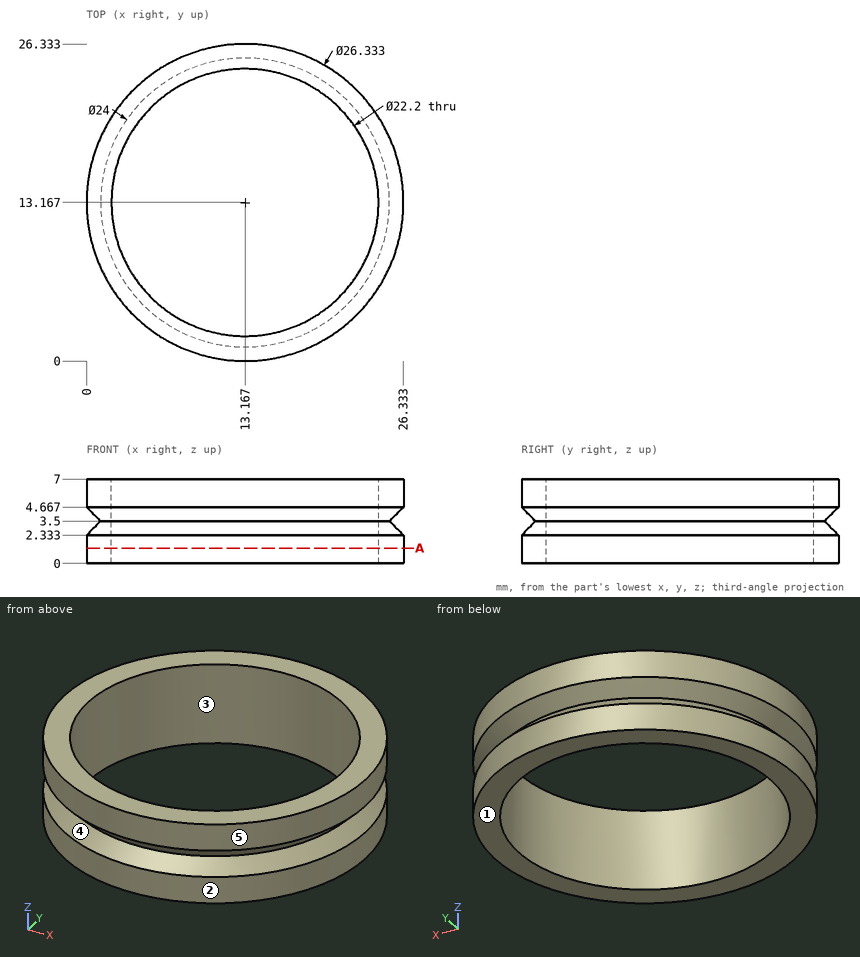
The drawing under review shows one solid part. Ordinate dimensions are in mm from its lowest x, y, z. A direction names the side the tool comes from. Coordinates: 2 decimals unless noted, no trailing zeros. Loops run counter-clockwise (first coordinate to the right, second up) from the corner with the lowest first, then second, coordinate; pieces in that order, holes last. Notation, with made-up numbers: (24, -6.75) - (34, -6.75) arc R10 cw to (34, -0.75) - close; hole circle Ø9 at (5, -1). An arc over 180 degrees is marked (long way). Use CSV: the item, a comma, the result in double quotes. Start each with the question number.
1. Clearance check with flat-ended pins moving along their axes: pin 1 (4 mm diameter, centred on x = 16.5, z = 5.5, fed in from -Y); pin 2 (3 mm diameter, centred on y = 23, z = 5.5, fed in from -X); pin 3 (2 mm diameter, centred on x = 5.5, z = 2, fed in from -Y); pin 4 (8 mm diameter, centred on x = 14.5, y = 6.5, fed in from -Z). State where each tip first meets the part, or that it passes through.
2. Add section A-A on z = 1.25. Give the boundary of the cut face in (x, y).
3. To check wall thickness, follow probe 1 along Y at (x, z) = (13.5, 5) (1 decimal); probe 2 along X at (y, z) = (15.25, 4) (1 decimal). State the ranges of each line that lie inside material, in increasing order.
4. For the marked faces 4 and 5, list the 3-axis set-ups (+Z, -Z, +X, -X, +Y, -Y) from which the entire face can be reached by the end or side of a thin tool; tool diameter is ignored.
5. Mouldability with a two-part tool opening along Y and no side actions: class the marked faces 1, 2 and 3 as released by +Y, released by -Y, zero draft, split by the parting line, or undercut.
Resolved:
1,pin 1,"y = 0.07"
1,pin 2,"x = 2.97"
1,pin 3,"y = 1.81"
1,pin 4,"through"
2,outline,"circle Ø26.33 at (13.17, 13.17); hole circle Ø22.2 at (13.17, 13.17)"
3,probe 1,"0 to 2.1, 24.3 to 26.3"
3,probe 2,"0.8 to 2.3, 24.1 to 25.5"
4,face 4,"none"
4,face 5,"+Z, -Z"
5,face 1,"zero draft"
5,face 2,"split by the parting line"
5,face 3,"undercut"
